Autodesk Inventor part; units mm, degrees
ref_plane "WorkPlane2" through (0, 0, 0) normal (0, 0, 1) x (1, 0, 0)
ref_plane "Work Plane2" through (0, 0, -3.9) normal (0, 0, 1) x (1, 0, 0)
ref_plane "WorkPlane3" through (0, 0, 7) normal (0, 0, 1) x (1, 0, 0)
ref_plane "WorkPlane2" through (0, 0, 0) normal (0, 0, 1) x (1, 0, 0)
sketch "Sketch1" plane through (0, 0, 0) normal (1, 0, 0) x (0, 1, 0)
  point P0 (0, 0)
ref_plane "Work Plane2" through (0, 0, -3.9) normal (0, 0, 1) x (1, 0, 0)
ref_plane "WorkPlane3" through (0, 0, 7) normal (0, 0, 1) x (1, 0, 0)
sketch "Sketch2" plane through (0, 0, 0) normal (0, 1, 0) x (-1, 0, 0)
  point P0 (0, 0)
sketch "Sketch3" plane through (0, 0, 0) normal (1, 0, 0) x (0, 1, 0)
  line L0 (2.5, -5.5) -> (2.1, -4.7)
  line L1 (2.5, -26.2) -> (2.5, -5.5)
  line L2 (0, -26.2) -> (2.5, -26.2)
  line L3 (0, 0) -> (0, -26.2)
  arc A0 (4.65, -1.2) -> (0, 0) centre (0, -9.6094) ccw
  line L4 (4.65, -1.35) -> (4.65, -1.2)
  line L5 (2.1, -3.9) -> (4.65, -1.35)
  line L6 (2.1, -4.7) -> (2.1, -3.9)
  line L7 (0, -31.6445) -> (0, 31.6445) construction
  line L8 (0, -31.6445) -> (0, 31.6445)
  line L9 (0, -44.3023) -> (0, 44.3023)
  dimension "d2" = 2.5
  dimension "d4" = 2.1
  dimension "d6" = 0.8
  dimension "d8" = 2.7
  dimension "d10" = 135
  dimension "d12" = 4.65
  dimension "d14" = 0
  dimension "d16" = 1.2
  dimension "d18" = 25
  dimension "d22" = 20.7
revolve "Revolution1" add sketch "Sketch3" angle 360 about axis through (0, 0, -31.6445) along (0, 0, 1)
fillet "Fillet1" radius 1.3 1 edges at (0, -2.1, -3.9)
sketch "Sketch4" plane through (0, 0, 0) normal (0, 1, 0) x (-1, 0, 0)
  line L0 (0, 0) -> (-2.7, 0)
  line L1 (0, -2.25) -> (0, 0)
  line L2 (-2.7, 0) -> (-0.45, -2.25)
  line L3 (0, -11.5313) -> (0, 1.9219)
  arc A0 (4.65, -1.2) -> (-4.65, -1.2) centre (0, -9.6094) ccw
  line L4 (0, -2.25) -> (-0.45, -2.25)
  point P0 (0, -2.7)
  dimension "d30" = 45
  dimension "d33" = 5.4
  dimension "d34" = 0.45
  dimension "d35" = 90
extrude "Extrusion1" cut sketch "Sketch4" along normal mid plane 0.9
pattern_circular "PolarArray1" count 4 over 360 about axis through (0, 0, -10) along (0, 0, 1) of "Extrusion1"
thread "Thread1"
ref_plane "MSC_PF1" through (0, 0, 0) normal (1, 0, 0) x (0, 1, 0)
ref_plane "MSC_PT1" through (0, 4.65, -1.35) normal (0, 0, -1) x (-1, 0, 0)
equation "\"d2\" = 0.5 * NND"
equation "\"d4\" = 0.5 * msp_mdtds"
equation "\"d6\" = msp_x"
equation "\"d8\" = ParK"
equation "\"d12\" = 0.5 * Dk"
equation "\"d16\" = ParF"
equation "\"d18\" = NLG"
equation "\"d22\" = b"
equation "\"d24\" = r"
equation "\"d33\" = M"
equation "\"d31\" = 0.166667 * M"
equation "\"d39\" = b"
equation "\"PTC\" = 0.8"
equation "\"msp_x\" = PTC"
equation "\"NLG\" = 25"
equation "\"NND\" = 5"
equation "\"ParK\" = 2.7"
equation "\"r\" = 1.3"
equation "\"msp_mdtds\" = NND - PTC"
equation "\"b\" = 20.7"
equation "\"Dk\" = 9.3"
equation "\"ParF\" = 1.2"
equation "\"M\" = 5.4"
equation "\"ParA\" = 1.6"
equation "\"THREADDIA\" = NND"
equation "\"TEMPLATE\" = 1.2345"
properties part number "ISO 7047 - M5x25 - 4.8 - H" material "Steel"
Check sheet for the modelled part. Datum: model origin and axes. Units: mm. A direction names the side the tool comes from. Round coordinates to 2 decimals unless told otherwise and drop trailing zeros. Order: outer loops, then holes, each group sorted by start corner. A loop starts at its lowest first (then second) coordinate and runs counter-clockwise, first axis right, second up.
1) Go/stop test with flat-tipped pins: pin 1 Ø1.5 at (x, z) = (0, -10) entering from +Y; pin 2 Ø5 at (x, y) = (2.5, 1) entering from +Z; pin 3 Ø2 at (x, z) = (1.5, -1) entering from +Y; pin 4 Ø1.6 at (y, z) = (1.5, -1.5) entering from -X. Record where each tip stops, or that it passes through.
2) Scan lines: line 1 (X direction, y = -0.25, z = -14.5); line 2 (X direction, y = 0, z = -1.25). Record each from-to range of solid material in increasing order.
3) Tool access check on faces 1 (the cylindrical face through (2.44, -0.54, -15.71)), 2 (the flat face through (0, 0, -26.2)), 3 (the flat face through (0, 0, -2.25)). Record the directions out of +Z, -Z, +X, -X, +Y, -Y that give a thin tool (end or side, any length) a straight path to the whole face; none if there is none.
4) Section check A-A (z = -8). Record the boundary of the cut face in (x, y), and give its area (3 significant figures).
Result:
1. pin 1: stops at y = 2.5
1. pin 2: stops at z = -0.02
1. pin 3: stops at y = 4.62
1. pin 4: stops at x = -4.59
2. line 1: x = -2.49 to 2.49
2. line 2: x = -4.65 to -1.45, 1.45 to 4.65
3. face 1: -Z
3. face 2: -Z, +X, -X, +Y, -Y
3. face 3: +Z
4. outline: circle Ø5 at (0, 0)
4. area: 19.6 mm2
